The model under review builds one solid part; all positions refer to its coordinate system, in mm. A direction names the side the tool comes from. Coordinates: 2 decimals unless noted, no trailing zeros. Loops run counter-clockwise (first coordinate to the right, second up) from the corner with the lowest first, then second, coordinate; pieces in that order, holes last. Notation, with made-up numbers: M 16,68 L 36,68 A20 cw 36,106 Z; hole C 61.25,1.5 d4. An arc over 180 degrees is marked long. Return JSON: item names as keys, results as strings.
```python
from build123d import *

# Parameters (mm, degrees)
BOSS_EXTRUDE1_DEPTH      = 7.5
BOSS_EXTRUDE1_DEPTH_BACK = 7.5
TAP_DRILL_FOR_M8_TAP1_D  = 6.8


with BuildPart() as part:
    # Sketch1 → Boss-Extrude1 (new, two sides: drawn at the far end of the back side and taken through both)
    with BuildSketch(Plane.XY.offset(-BOSS_EXTRUDE1_DEPTH_BACK)):
        with BuildLine():
            Line((-33, 0), (-16, 0))
            ThreePointArc((-16, 0), (0, -16), (16, 0))
            Line((16, 0), (33, 0))
            Line((33, 0), (33, -17))
            Line((33, -17), (18.33030278, -17))
            ThreePointArc((18.33030278, -17), (0, -25), (-18.33030278, -17))
            Line((-18.33030278, -17), (-33, -17))
            Line((-33, -17), (-33, 0))
        make_face()
    extrude(amount=BOSS_EXTRUDE1_DEPTH + BOSS_EXTRUDE1_DEPTH_BACK)

    # Tap Drill for M8 Tap1 (through all)
    with Locations(Plane(origin=(0, -17, 0), x_dir=(-1, 0, 0), z_dir=(0, -1, 0))):
        with Locations((26.25, 0), (-26.25, 0)):
            Hole(TAP_DRILL_FOR_M8_TAP1_D / 2)


solid = part.part
```
1. The part is to be moulded in two halves that separate along Z. For faces 3 (the face through (0, -18, -7.5)), 4 (the face through (22.5, -17, -0.1)), 5 (the face through (-23, -8, 1)), say which applies: released by +Z, released by -Z, zero draft, split by the parting line, or undercut.
Check values:
{"face 3": "released by -Z", "face 4": "zero draft", "face 5": "undercut"}
2. Insertion check: pin 1 Ø3 at (x, z) = (-17, 2.5) entering from -Y; pin 2 Ø4.5 at (x, z) = (-23, 3) entering from -Y; pin 3 Ø6 at (x, z) = (26.25, 0) entering from -Y. Each pin has a flat end and moves straight along its axis. Give the tip position at first contact, or say it passes through.
Check values:
{"pin 1": "y = -19.62", "pin 2": "y = -17", "pin 3": "through"}
3. Add section A-A on y = -13. Give the boundary of the cut face in (x, z).
Check values:
{"outline": "M -33,-7.5 L -9.33,-7.5 L -9.33,7.5 L -33,7.5 Z; M 9.33,-7.5 L 33,-7.5 L 33,7.5 L 9.33,7.5 Z; hole C -26.25,0 d6.8; hole C 26.25,0 d6.8"}
4. Machinability: for faces 1 (the face through (-22, -17, 0)), 2 (the face through (-22.7, 0, -0.1)), which of the approach directions +Z, -Z, +X, -X, +Y, -Y give a long, thin tool a straight path to every point of the face, cutting with its end or side? Answer none if there is none.
Check values:
{"face 1": "+Z, -Z, -X, -Y", "face 2": "+Z, -Z, +X, -X, +Y"}
5. Add section C-C on z = -1.75. Give the boundary of the cut face in (x, y), plus the area to 3 significant figures.
Check values:
{"outline": "M -33,-17 L -29.17,-17 L -29.17,0 L -33,0 Z; M -23.33,-17 L -18.33,-17 A25 ccw 18.33,-17 L 23.33,-17 L 23.33,0 L 16,0 A16 cw -16,0 L -23.33,0 Z; M 29.17,-17 L 33,-17 L 33,0 L 29.17,0 Z", "area": "724 mm²"}
6. Add section D-D on z = -5.5. Give the boundary of the cut face in (x, y).
Check values:
{"outline": "M -33,-17 L -18.33,-17 A25 ccw 18.33,-17 L 33,-17 L 33,0 L 16,0 A16 cw -16,0 L -33,0 Z"}
7. To check wall thickness, follow line 1 (Z direction, x = 26.25, y = -6.75); line 2 (Y direction, x = 20, z = 6.5); line 3 (X direction, y = -10.75, z = 1.75). State the ranges of each line that lie inside material, in increasing order.
Check values:
{"line 1": "-7.5 to -3.4, 3.4 to 7.5", "line 2": "-17 to 0", "line 3": "-33 to -29.17, -23.33 to -11.85, 11.85 to 23.33, 29.17 to 33"}
8. Add section B-B on x = -26.25. Give the boundary of the cut face in (y, z), plus the area to 3 significant figures.
Check values:
{"outline": "M -17,-7.5 L 0,-7.5 L 0,-3.4 L -17,-3.4 Z; M -17,3.4 L 0,3.4 L 0,7.5 L -17,7.5 Z", "area": "139 mm²"}
